Verification items for the finished model (mm, model axes). A direction names the side the tool comes from. Round coordinates to 2 decimals unless told otherwise and drop trailing zeros. Order: outer loops, then holes, each group sorted by start corner. A loop starts at its lowest first (then second) coordinate and runs counter-clockwise, first axis right, second up. Notation, with made-up numbers: (50.5, 65.5) -> (74.5, 65.5) arc R3 cw to (74.5, 69.5) -> close; hole circle Ø9 at (36.5, 18). An arc over 180 degrees is marked (long way). Put each result on its own line as item: value.
```python
from build123d import *

# Parameters (mm, degrees)
SKETCH_1_R          = 45
EXTRUDE_1_DEPTH     = 15
SKETCH_2_R          = 20
EXTRUDE_2_DEPTH     = 65
SKETCH_4_R          = 10.9
CUT_EXTRUDE_4_DEPTH = 52
EXTRUDE_START       = 8
SKETCH_5_R          = 35
SKETCH_5_R_2        = 10.9
EXTRUDE_5_DEPTH     = 8
CHAMFER_3_SIZE      = 2
CHAMFER_4_SIZE      = 6
CHAMFER_4_SIZE2     = 10.392304845
SKETCH_6_R          = 7
CUT_EXTRUDE_8_DEPTH = 4
CUT_EXTRUDE_1_REACH = 91.549
SKETCH_7_R          = 3


with BuildPart() as part:
    # Эскиз1 → Вытянуть1 (new body)
    with BuildSketch(Plane(origin=(0, 0, 0), x_dir=(1, 0, 0), z_dir=(0, 1, 0))):
        with Locations(Location((0, 0, 0), (0, 0, 270))):
            Circle(SKETCH_1_R)
        with BuildLine():
            Line((-2, -6.708203932), (-2, -8.85))
            Line((-2, -8.85), (2.5, -8.85))
            Line((2.5, -8.85), (2.5, -6.538348415))
            ThreePointArc((2.5, -6.538348415), (-0.264031673, 6.995018747), (-2, -6.708203932))
        make_face(mode=Mode.SUBTRACT)
    extrude(amount=EXTRUDE_1_DEPTH)

    # Эскиз2 → Вытянуть2 (add)
    with BuildSketch(Plane(origin=(0, 15, 0), x_dir=(1, 0, 0), z_dir=(0, 1, 0))):
        with Locations(Location((0, 0, 0), (0, 0, 270))):
            Circle(SKETCH_2_R)
    extrude(amount=EXTRUDE_2_DEPTH)

    # Эскиз4 → Вытянуть4 (cut)
    with BuildSketch(Plane(origin=(0, 80, 0), x_dir=(1, 0, 0), z_dir=(0, 1, 0))):
        with Locations(Location((0, 0, 0), (0, 0, 270))):
            Circle(SKETCH_4_R)
    extrude(amount=-CUT_EXTRUDE_4_DEPTH, mode=Mode.SUBTRACT)

    # Эскиз5 → Вытянуть5 (add)
    with BuildSketch(Plane(origin=(0, 55, 0), x_dir=(-1, 0, 0), z_dir=(0, 1, 0)).offset(EXTRUDE_START)):
        with Locations(Location((0, 0, 0), (0, 0, 90))):
            Circle(SKETCH_5_R)
        with Locations(Location((0, 0, 0), (0, 0, 90))):
            Circle(SKETCH_5_R_2, mode=Mode.SUBTRACT)
    extrude(amount=-EXTRUDE_5_DEPTH)

    # Фаска3
    chamfer_3_edges = [part.edges().sort_by_distance(p)[0] for p in [
        (0, 55, -20),
        (0, 63, -20),
    ]]
    chamfer(chamfer_3_edges, length=CHAMFER_3_SIZE)

    # Фаска4
    chamfer_4_edges = [part.edges().sort_by_distance(p)[0] for p in [
        (0, 15, -20),
    ]]
    chamfer_4_side = [part.faces().sort_by_distance(p)[0] for p in [
        (0, 15, -43.727207794),
    ]]
    chamfer(chamfer_4_edges, length=CHAMFER_4_SIZE, length2=CHAMFER_4_SIZE2, reference=chamfer_4_side[0])

    # Эскиз6 → Вытянуть8 (cut)
    with BuildSketch(Plane.XZ.offset(-15)):
        with Locations(Location((0, 0, 0), (0, 0, 270))):
            Circle(SKETCH_6_R)
    extrude(amount=-CUT_EXTRUDE_8_DEPTH, mode=Mode.SUBTRACT)

    # Эскиз7 → Вырез-Вытянуть1 (cut, up to next)
    with BuildSketch(Plane(origin=(0, 63, 0), x_dir=(1, 0, 0), z_dir=(0, 1, 0)), mode=Mode.PRIVATE) as cut_extrude_1_sk1:
        with Locations(Location((-28.154160791, -0.499908421, 0), (0, 0, 270))):
            Circle(SKETCH_7_R)
    cut_extrude_1_tool1 = extrude(cut_extrude_1_sk1.sketch, amount=-CUT_EXTRUDE_1_REACH, mode=Mode.PRIVATE) & part.part
    # Эскиз7 → Вырез-Вытянуть1 (cut, up to next)
    with BuildSketch(Plane(origin=(0, 63, 0), x_dir=(1, 0, 0), z_dir=(0, 1, 0)), mode=Mode.PRIVATE) as cut_extrude_1_sk2:
        with Locations(Location((-14.510013788, 24.132264256, 0), (0, 0, 270))):
            Circle(SKETCH_7_R)
    cut_extrude_1_tool2 = extrude(cut_extrude_1_sk2.sketch, amount=-CUT_EXTRUDE_1_REACH, mode=Mode.PRIVATE) & part.part
    # Эскиз7 → Вырез-Вытянуть1 (cut, up to next)
    with BuildSketch(Plane(origin=(0, 63, 0), x_dir=(1, 0, 0), z_dir=(0, 1, 0)), mode=Mode.PRIVATE) as cut_extrude_1_sk3:
        with Locations(Location((13.644147003, 24.632172678, 0), (0, 0, 270))):
            Circle(SKETCH_7_R)
    cut_extrude_1_tool3 = extrude(cut_extrude_1_sk3.sketch, amount=-CUT_EXTRUDE_1_REACH, mode=Mode.PRIVATE) & part.part
    # Эскиз7 → Вырез-Вытянуть1 (cut, up to next)
    with BuildSketch(Plane(origin=(0, 63, 0), x_dir=(1, 0, 0), z_dir=(0, 1, 0)), mode=Mode.PRIVATE) as cut_extrude_1_sk4:
        with Locations(Location((28.154160791, 0.499908421, 0), (0, 0, 270))):
            Circle(SKETCH_7_R)
    cut_extrude_1_tool4 = extrude(cut_extrude_1_sk4.sketch, amount=-CUT_EXTRUDE_1_REACH, mode=Mode.PRIVATE) & part.part
    # Эскиз7 → Вырез-Вытянуть1 (cut, up to next)
    with BuildSketch(Plane(origin=(0, 63, 0), x_dir=(1, 0, 0), z_dir=(0, 1, 0)), mode=Mode.PRIVATE) as cut_extrude_1_sk5:
        with Locations(Location((14.510013788, -24.132264256, 0), (0, 0, 270))):
            Circle(SKETCH_7_R)
    cut_extrude_1_tool5 = extrude(cut_extrude_1_sk5.sketch, amount=-CUT_EXTRUDE_1_REACH, mode=Mode.PRIVATE) & part.part
    # Эскиз7 → Вырез-Вытянуть1 (cut, up to next)
    with BuildSketch(Plane(origin=(0, 63, 0), x_dir=(1, 0, 0), z_dir=(0, 1, 0)), mode=Mode.PRIVATE) as cut_extrude_1_sk6:
        with Locations(Location((-13.644147003, -24.632172678, 0), (0, 0, 270))):
            Circle(SKETCH_7_R)
    cut_extrude_1_tool6 = extrude(cut_extrude_1_sk6.sketch, amount=-CUT_EXTRUDE_1_REACH, mode=Mode.PRIVATE) & part.part
    add(cut_extrude_1_tool1.solids().sort_by_distance((-28.154161, 63, 0.499908))[0], mode=Mode.SUBTRACT)
    add(cut_extrude_1_tool2.solids().sort_by_distance((-14.510014, 63, -24.132264))[0], mode=Mode.SUBTRACT)
    add(cut_extrude_1_tool3.solids().sort_by_distance((13.644147, 63, -24.632173))[0], mode=Mode.SUBTRACT)
    add(cut_extrude_1_tool4.solids().sort_by_distance((28.154161, 63, -0.499908))[0], mode=Mode.SUBTRACT)
    add(cut_extrude_1_tool5.solids().sort_by_distance((14.510014, 63, 24.132264))[0], mode=Mode.SUBTRACT)
    add(cut_extrude_1_tool6.solids().sort_by_distance((-13.644147, 63, 24.632173))[0], mode=Mode.SUBTRACT)


solid = part.part
```
Item 1: Material ranges on line 1 along X through (y, z) = (9, 0); line 2 along Y through (x, z) = (31, 13); line 3 along X through (y, z) = (56.5, -26), recorded low to high.
Geometry check:
line 1: -45 to -7, 7 to 45
line 2: 0 to 15, 55 to 63
line 3: -23.43 to -16.86, -12.16 to 10.97, 16.31 to 23.43
Item 2: Depth check by flat-ended pin: pin 1 Ø1.8 at (y, z) = (5.5, 8) entering from -X; pin 2 Ø10 at (x, z) = (-27.5, -3) entering from +Y; pin 3 Ø5.5 at (x, z) = (13.64, -24.63) entering from +Y; pin 4 Ø1 at (x, y) = (-21, 47) entering from -Z. Enter the tip coordinate at first touch or a pass-through.
Geometry check:
pin 1: x = -44.44
pin 2: y = 63
pin 3: y = 16.03
pin 4: through
Item 3: Release check for a two-part mould opening along X. For faces 4 (the face through (-19.524, 39.003, -4.336)), 5 (the face through (-9, 0, -1)), 6 (the face through (2.5, 7, 8)) record: pulls with the +X half, pulls with the -X half, needs draft (parallel to the pull), parting line crosses it, or undercut.
Geometry check:
face 4: parting line crosses it
face 5: needs draft
face 6: undercut
Item 4: Sectioned sample at A-A, the plane z = 30.5. Record the boundary of the cut face in (x, y), then the cut area to 3 significant figures.
Geometry check:
outline: (-33.09, 0) -> (33.09, 0) -> (33.09, 15) -> (-33.09, 15) -> close; (-17.17, 55) -> (17.17, 55) -> (17.17, 63) -> (-17.17, 63) -> close
area: 1,270 mm2
Item 5: Sectioned sample at D-D, the plane z = 0. Give the number of separate pieces and of enclosed holes in the cut face, then the cut area to 3 significant figures.
Geometry check:
separate pieces: 3
enclosed holes: 0
area: 2,770 mm2
Item 6: Tool access check on faces 1 (the face through (0, 7, 8.85)), 2 (the face through (-13.512, 59.056, 21.635)), 3 (the face through (-19, 15, 19)). Record the directions out of +Z, -Z, +X, -X, +Y, -Y that give a thin tool (end or side, any length) a straight path to the whole face; none if there is none.
Geometry check:
face 1: -Y
face 2: +Y
face 3: none
Item 7: Sectioned sample at C-C, the plane y = 66.5. Record the boundary of the cut face in (x, z), then the cut area to 3 significant figures.
Geometry check:
outline: circle Ø40 at (0, 0); hole circle Ø21.8 at (0, 0)
area: 883 mm2
